```python
from build123d import *

# Parameters (mm, degrees)
SKETCH002_R = 7.3
PAD_DEPTH   = 8


with BuildPart() as part:
    # Sketch002 → Pad (new body)
    with BuildSketch(Plane(origin=(0, 0, 0), x_dir=(1, 0, 0), z_dir=(0, 0, -1))):
        with Locations((-32, 0)):
            Circle(SKETCH002_R)
        Polygon((-34.944486, 5.1), (-37.888973, 0), (-34.944486, -5.1), (-29.055514, -5.1), (-26.111027, 0), (-29.055514, 5.1), align=None, mode=Mode.SUBTRACT)
    extrude(amount=PAD_DEPTH)


solid = part.part
```
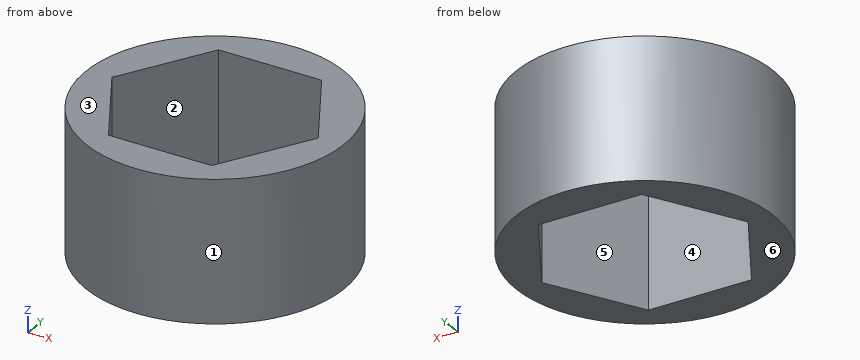
Here's how the part is built. I have some questions about the finished solid (model axes, mm). Face numbers are marked on the shaded views. A direction names the side the tool comes from. Give positions to 0.01 mm unless a question says otherwise; leave off trailing zeros. Loops run counter-clockwise (first coordinate to the right, second up) from the corner with the lowest first, then second, coordinate; pieces in that order, holes last. Notation, with made-up numbers: (63.5, 9.25) -> (100.5, 9.25) arc R22 cw to (100.5, 30.25) -> close; hole circle Ø6 at (34, 51). An arc over 180 degrees is marked (long way). Use one line per item in the form item = value. Start each with the question number.
1) Thinking about a two-plate mould opening in X: for the marked faces 1, 2, 3 and 4, which applies, +X half, -X half, draft (parallel to the pull), parting line (faces both ways), or undercut?
2) Imagine slicing it at B-B (z = -5). Please give me the cut outline in (x, y).
3) Imagine slicing it at A-A (x = -32). Please give me the cut outline in (y, z).
4) For P1, Ø1.5, axis at y = -2.5, z = -1.5, coming from the -X side; P2, Ø2, axis at x = -35.5, z = -4.5, coming from the +Y side; P3, Ø1, axis at x = -28.5, y = 2, coming from the +Z side; P4, Ø1, axis at y = -4, z = -5.5, coming from the +X side, each with a flat end and sliding along its axis, tell me the tip position at first contact or that it passes through.
5) Please list where these lines run through material, in increasing order: line 1 along Y through (x, z) = (-30.75, -1.25); line 2 along X through (y, z) = (4.5, -4.5); line 3 along Y through (x, z) = (-27, -0.75).
6) Imagine slicing it at C-C (y = -0.5). Please give me the cut outline in (x, z).
7) Which directions (+Z, -Z, +X, -X, +Y, -Y) give clear straight access to the entire face, cutting with the end or side of a thin tool? Please do the marked faces 5 and 6.
Check values:
q1.face_1 = parting line
q1.face_2 = undercut
q1.face_3 = draft
q1.face_4 = undercut
q2.outline = circle Ø14.6 at (-32, 0); hole (-37.89, 0) -> (-34.94, -5.1) -> (-29.06, -5.1) -> (-26.11, 0) -> (-29.06, 5.1) -> (-34.94, 5.1) -> close
q3.outline = (-7.3, -8) -> (-5.1, -8) -> (-5.1, 0) -> (-7.3, 0) -> close; (5.1, -8) -> (7.3, -8) -> (7.3, 0) -> (5.1, 0) -> close
q4.P1 = -39.09
q4.P2 = 6.86
q4.P3 = through
q4.P4 = -25.59
q5.line_1 = -7.19 to -5.1, 5.1 to 7.19
q5.line_2 = -37.75 to -35.29, -28.71 to -26.25
q5.line_3 = -5.32 to -1.54, 1.54 to 5.32
q6.outline = (-39.28, -8) -> (-37.6, -8) -> (-37.6, 0) -> (-39.28, 0) -> close; (-26.4, -8) -> (-24.72, -8) -> (-24.72, 0) -> (-26.4, 0) -> close
q7.face_5 = +Z, -Z
q7.face_6 = -Z, +X, -X, +Y, -Y
